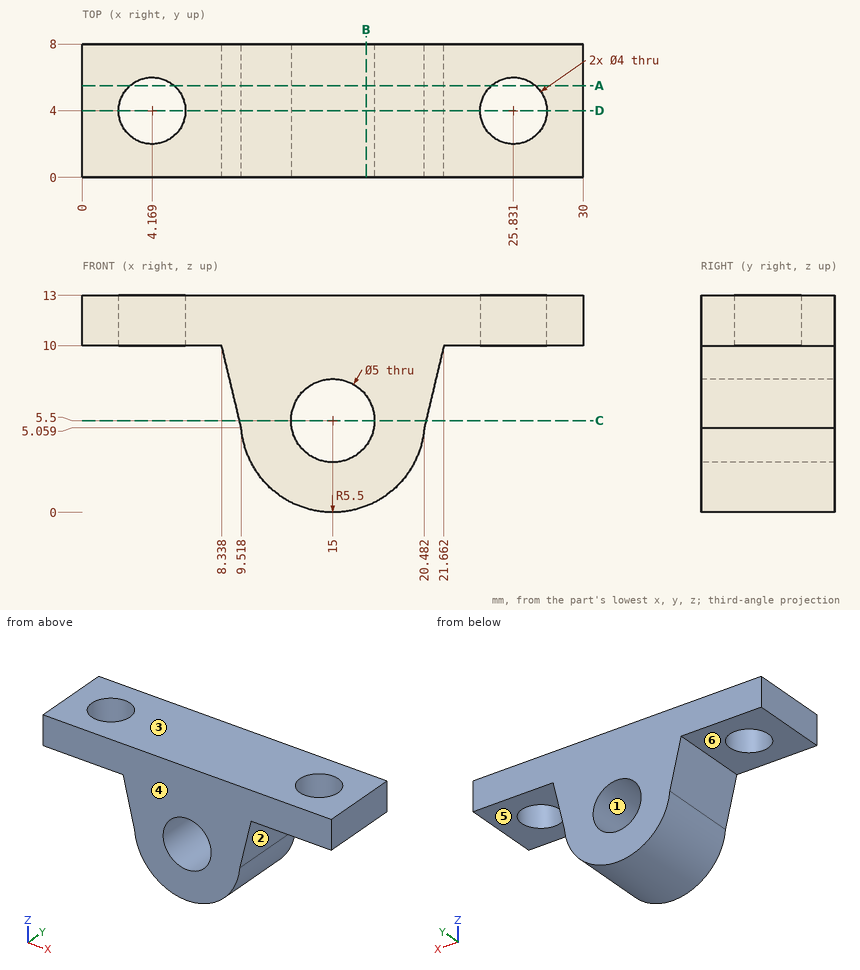
Here's the drawing with two shaded views (mm, measured from the low corner). I have some questions. A direction names the side the tool comes from. Give positions to 0.01 mm unless a question says otherwise; leave off trailing zeros. Loops run counter-clockwise (first coordinate to the right, second up) from the corner with the lowest first, then second, coordinate; pieces in that order, holes last. Notation, with made-up numbers: M -4,36.25 L 41,36.25 A12 ccw 41,55.25 Z; hole C -21,-25 d4. An arc over 180 degrees is marked long. One line per item, written item: value.
(1) We'd pull the mould along X, two halves only. Please class the marked faces 1, 2 and 3: released by +X, released by -X, zero draft, split by the parting line, or undercut.
Returned:
face 1: undercut
face 2: released by +X
face 3: zero draft
(2) Suppose I cut it at D-D on y = 4. List the corners of the cut face in (x, z) for me.
Returned:
outline: M 0,10 L 2.17,10 L 2.17,13 L 0,13 Z; M 6.17,10 L 8.34,10 L 9.52,5.06 A5.5 ccw 20.48,5.06 L 21.66,10 L 23.83,10 L 23.83,13 L 6.17,13 Z; M 27.83,10 L 30,10 L 30,13 L 27.83,13 Z; hole C 15,5.5 d5
(3) Which directions (+Z, -Z, +X, -X, +Y, -Y) give clear straight access to the entire face, cutting with the end or side of a thin tool? Please do the marked faces 4, 5 and 6.
Returned:
face 4: +Z, -Z, +X, -X, -Y
face 5: -Z, +X, +Y, -Y
face 6: -Z, -X, +Y, -Y
(4) I need wall thicknesses on line 1 (Z direction, x = 13.75, y = 7.5) (1 decimal); line 2 (X direction, y = 5, z = 6); line 3 (X direction, y = 1.5, z = 5.5). Which ranges of each line are inside material? Lowest first, please.
Returned:
line 1: 0.1 to 3.3, 7.7 to 13
line 2: 9.29 to 12.55, 17.45 to 20.71
line 3: 9.41 to 12.5, 17.5 to 20.59
(5) Suppose I cut it at A-A on y = 5.5. List the corners of the cut face in (x, z) for me.
Returned:
outline: M 0,10 L 2.85,10 L 2.85,13 L 0,13 Z; M 5.49,10 L 8.34,10 L 9.52,5.06 A5.5 ccw 20.48,5.06 L 21.66,10 L 24.51,10 L 24.51,13 L 5.49,13 Z; M 27.15,10 L 30,10 L 30,13 L 27.15,13 Z; hole C 15,5.5 d5
(6) Suppose I cut it at C-C on z = 5.5. List the corners of the cut face in (x, y) for me.
Returned:
outline: M 9.41,0 L 12.5,0 L 12.5,8 L 9.41,8 Z; M 17.5,0 L 20.59,0 L 20.59,8 L 17.5,8 Z
(7) Will this pin go through, and if not, where does the flat tip stop? pin 1 (4 mm diameter, centred on x = 24, y = 4, fed in from -Z).
Returned:
pin 1: z = 10
(8) Suppose I cut it at B-B on x = 17. List the corners of the cut face in (y, z) for me, plus the area to 3 significant figures.
Returned:
outline: M 0,0.38 L 8,0.38 L 8,4 L 0,4 Z; M 0,7 L 8,7 L 8,13 L 0,13 Z
area: 77.0 mm^2
